Check sheet for the modelled part. Datum: model origin and axes. Units: mm. Face numbers are marked on the shaded views. A direction names the side the tool comes from. Give positions to 0.01 mm unless a question says otherwise; leave off trailing zeros. Loops run counter-clockwise (first coordinate to the right, second up) from the corner with the lowest first, then second, coordinate; pieces in that order, holes last. Notation, with made-up numbers: (25.5, -32.75) -> (58.5, -32.75) arc R16 ccw to (58.5, -14.75) -> close; hole circle Ø10 at (4, -13). An arc over 180 degrees is marked (long way). Answer as CSV lines item,"result". Start each with the question number.
(1) Gauge pin test, flat ends, axial feed: pin 1 Ø2 at (y, z) = (-8, 2.5) entering from -X; pin 2 Ø1.2 at (x, z) = (0.5, 0) entering from +Y; pin 3 Ø2 at (y, z) = (-6.5, -1.5) entering from -X; pin 4 Ø2 at (x, z) = (-1, 2) entering from -Y. Record the tip position at first contact, or that the pin passes through.
(2) Access from +Z, -Z, +X, -X, +Y, -Y to the whole of each face (thin tool, end or side, straight path). Record for the marked faces 5 and 6.
(3) Section check B-B on y = -9.75. Enter the section's corners in (x, z).
(4) Material ranges on line 1 (Y direction, x = 0, z = 0.25); line 2 (Y direction, x = 2, z = -2); line 3 (X direction, y = 2.75, z = -0.75), recorded low to high. Write a range as from..to.
(5) Section check A-A on x = 0. Enter the section's corners in (y, z).
(6) Release check for a two-part mould opening along Z. For the marked faces 1, 2, 3 and 4 record: pulls with the +Z half, pulls with the -Z half, needs draft (parallel to the pull), parting line crosses it, or undercut.
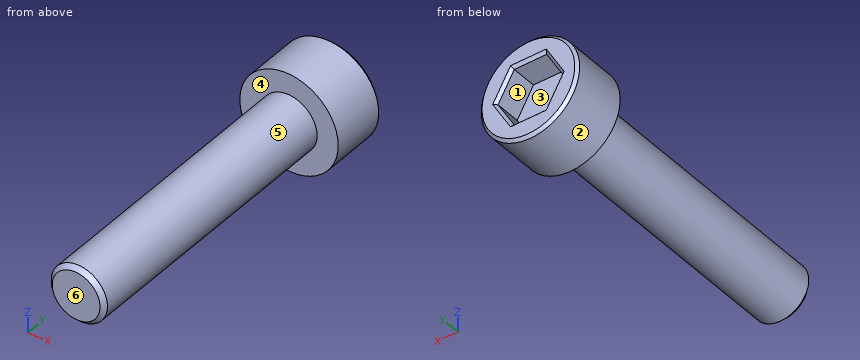
from build123d import *

# Parameters (mm, degrees)
SKETCH_1_R          = 3.5
EXTRUDE_1_DEPTH     = 4
SKETCH_2_R          = 2
EXTRUDE_2_DEPTH     = 20
CUT_EXTRUDE_1_DEPTH = 2
CHAMFER_1_SIZE      = 0.2
CHAMFER_2_SIZE      = 0.3


with BuildPart() as part:
    # 草图1 → 凸台-拉伸1 (new body)
    with BuildSketch(Plane(origin=(0, 0, 0), x_dir=(1, 0, 0), z_dir=(0, 1, 0))):
        Circle(SKETCH_1_R)
    extrude(amount=EXTRUDE_1_DEPTH)

    # 草图2 → 凸台-拉伸2 (add)
    with BuildSketch(Plane.XZ):
        Circle(SKETCH_2_R)
    extrude(amount=EXTRUDE_2_DEPTH)

    # 草图11 → 切除-拉伸1 (cut)
    with BuildSketch(Plane(origin=(0, 4, 0), x_dir=(1, 0, 0), z_dir=(0, 1, 0))):
        Polygon((1.154954177, 1.999853541), (-1.154446882, 2.000146427), (-2.309401058, 0.000292887), (-1.154954177, -1.999853541), (1.154446882, -2.000146427), (2.309401058, -0.000292887), align=None)
    extrude(amount=-CUT_EXTRUDE_1_DEPTH, mode=Mode.SUBTRACT)

    # 倒角1
    chamfer_1_edges = [part.edges().sort_by_distance(p)[0] for p in [
        (1.732177617, 4, -0.999780327),
        (0.000253647, 4, -1.999999984),
        (-1.73192397, 4, -1.000219657),
        (-1.732177617, 4, 0.999780327),
        (-0.000253647, 4, 1.999999984),
        (1.73192397, 4, 1.000219657),
        (-3.5, 4, 0),
    ]]
    chamfer(chamfer_1_edges, length=CHAMFER_1_SIZE)

    # 倒角2
    chamfer_2_edges = [part.edges().sort_by_distance(p)[0] for p in [
        (-2, -20, 0),
    ]]
    chamfer(chamfer_2_edges, length=CHAMFER_2_SIZE)


solid = part.part
Working result:
1,pin 1,"stops at x = -1.32"
1,pin 2,"stops at y = 2"
1,pin 3,"stops at x = -1.94"
1,pin 4,"stops at y = -20"
2,face 5,"-Y"
2,face 6,"+Z, -Z, +X, -X, -Y"
3,outline,"circle Ø4 at (0, 0)"
4,line 1,"y = -20..2"
4,line 2,"y = 0..4"
4,line 3,"x = -3.42..-1.88, 1.88..3.42"
5,outline,"(-20, -1.7) -> (-19.7, -2) -> (0, -2) -> (0, -3.5) -> (3.8, -3.5) -> (4, -3.3) -> (4, -2.2) -> (3.8, -2) -> (2, -2) -> (2, 2) -> (3.8, 2) -> (4, 2.2) -> (4, 3.3) -> (3.8, 3.5) -> (0, 3.5) -> (0, 2) -> (-19.7, 2) -> (-20, 1.7) -> close"
6,face 1,"undercut"
6,face 2,"parting line crosses it"
6,face 3,"undercut"
6,face 4,"needs draft"
